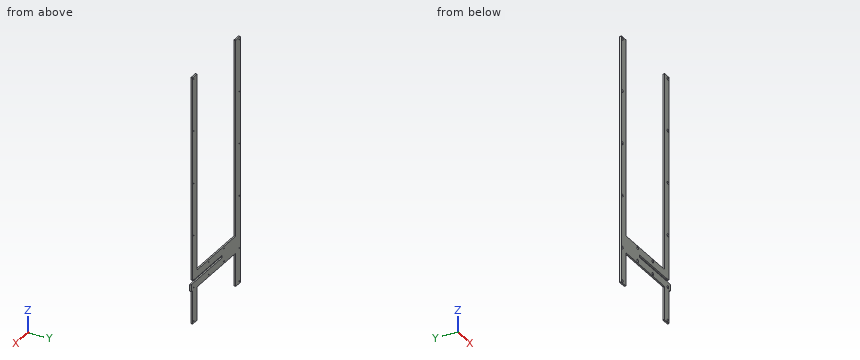
from build123d import *

# Parameters (mm, degrees)
BOSS_EXTRUDE1_DEPTH                                 = 9.525
SKETCH4_W                                           = 50.8
SKETCH4_H                                           = 200
BOSS_EXTRUDE2_DEPTH                                 = 9.525
CSK_FOR_1_4_FLAT_HEAD_MACHINE_SCREW_100_D           = 6.7564
CSK_FOR_1_4_FLAT_HEAD_MACHINE_SCREW_100_CSINK_D     = 17.6447958
CSK_FOR_1_4_FLAT_HEAD_MACHINE_SCREW_100_CSINK_ANGLE = 100
LPATTERN3_COUNT                                     = 2
LPATTERN3_PITCH                                     = 491.2
LPATTERN3_COUNT_DIR2                                = 5
LPATTERN3_PITCH_DIR2                                = 313.05
LPATTERN2_COUNT                                     = 3
LPATTERN2_PITCH                                     = 163.733333333
LPATTERN2_COUNT_DIR2                                = 2
LPATTERN2_PITCH_DIR2                                = 76.2
CSK_FOR_1_4_FLAT_HEAD_MACHINE_SCREW_2_D             = 6.7564
CSK_FOR_1_4_FLAT_HEAD_MACHINE_SCREW_2_CSINK_D       = 17.6447958
CSK_FOR_1_4_FLAT_HEAD_MACHINE_SCREW_2_CSINK_ANGLE   = 100
FILLET1_R                                           = 3.175
FILLET2_R                                           = 3.175


with BuildPart() as part:
    # Sketch1 → Boss-Extrude1 (new body)
    with BuildSketch(Plane(origin=(0, 0, 0), x_dir=(1, 0, 0), z_dir=(0, 1, 0))):
        Polygon((-258.3, 0), (-207.5, 0), (-207.5, 1176), (207.5, 1176), (207.5, 0), (258.3, 0), (258.3, 1215.514856628), (230.3, 1219.45), (-61.7, 1219.45), (-61.7, 1234.15), (271.3, 1234.15), (271.3, 1277.6), (-258.3, 1277.6), align=None)
    extrude(amount=BOSS_EXTRUDE1_DEPTH)

    # Sketch4 → Boss-Extrude2 (add)
    with BuildSketch(Plane.XZ):
        with Locations((-232.9, -1377.6)):
            Rectangle(SKETCH4_W, SKETCH4_H)
        with Locations((232.9, -1377.6)):
            Rectangle(SKETCH4_W, SKETCH4_H)
    extrude(amount=-BOSS_EXTRUDE2_DEPTH)

    # CSK for 1_4 Flat Head Machine Screw _100 (through all)
    with Locations(Plane.XZ):
        with Locations((-245.6, -1264.9)):
            csk_for_1_4_flat_head_machine_screw_100 = CounterSinkHole(CSK_FOR_1_4_FLAT_HEAD_MACHINE_SCREW_100_D / 2, CSK_FOR_1_4_FLAT_HEAD_MACHINE_SCREW_100_CSINK_D / 2, counter_sink_angle=CSK_FOR_1_4_FLAT_HEAD_MACHINE_SCREW_100_CSINK_ANGLE)

    # LPattern3: CSK for 1_4 Flat Head Machine Screw _100 2 × 5
    with Locations(*[(i * LPATTERN3_PITCH, 0, j * LPATTERN3_PITCH_DIR2) for i in range(LPATTERN3_COUNT) for j in range(LPATTERN3_COUNT_DIR2) if (i, j) != (0, 0)]):
        add(csk_for_1_4_flat_head_machine_screw_100, mode=Mode.SUBTRACT)

    # LPattern2: CSK for 1_4 Flat Head Machine Screw _100 3 × 2, 1 skipped
    with Locations(*[(i * LPATTERN2_PITCH, 0, j * LPATTERN2_PITCH_DIR2) for i in range(LPATTERN2_COUNT) for j in range(LPATTERN2_COUNT_DIR2) if (i, j) not in ((0, 0), (0, 1))]):
        add(csk_for_1_4_flat_head_machine_screw_100, mode=Mode.SUBTRACT)

    # CSK for 1_4 Flat Head Machine Screw  2 (through all)
    with Locations(Plane.XZ):
        with Locations((-245.6, -1464.9)):
            csk_for_1_4_flat_head_machine_screw_2 = CounterSinkHole(CSK_FOR_1_4_FLAT_HEAD_MACHINE_SCREW_2_D / 2, CSK_FOR_1_4_FLAT_HEAD_MACHINE_SCREW_2_CSINK_D / 2, counter_sink_angle=CSK_FOR_1_4_FLAT_HEAD_MACHINE_SCREW_2_CSINK_ANGLE)

    # Mirror1: CSK for 1_4 Flat Head Machine Screw  2 across plane
    add(csk_for_1_4_flat_head_machine_screw_2.mirror(Plane(origin=(0, 0, 0), x_dir=(0, 0, 1), z_dir=(1, 0, 0))), mode=Mode.SUBTRACT)

    # Fillet1
    fillet1_edges = [part.edges().sort_by_distance(p)[0] for p in [
        (258.3, 4.7625, 0),
        (207.5, 4.7625, 0),
        (-207.5, 4.7625, 0),
        (-258.3, 4.7625, 0),
        (207.5, 4.7625, -1176),
        (-207.5, 4.7625, -1176),
        (258.3, 4.7625, -1215.514856628),
        (271.3, 4.7625, -1234.15),
        (271.3, 4.7625, -1277.6),
        (-61.7, 4.7625, -1219.45),
        (-61.7, 4.7625, -1234.15),
    ]]
    fillet(fillet1_edges, radius=FILLET1_R)

    # Fillet2
    fillet2_edges = [part.edges().sort_by_distance(p)[0] for p in [
        (207.5, 4.7625, -1477.6),
        (258.3, 4.7625, -1477.6),
        (-258.3, 4.7625, -1477.6),
        (-207.5, 4.7625, -1477.6),
        (-207.5, 4.7625, -1277.6),
        (207.5, 4.7625, -1277.6),
        (258.3, 4.7625, -1277.6),
    ]]
    fillet(fillet2_edges, radius=FILLET2_R)


solid = part.part
The listing builds one solid part. Answer for the finished solid, in the listing's coordinates (mm). Round coordinates to 2 decimals unless told otherwise and drop trailing zeros. Write each loop counter-clockwise with the first axis right and the second up, starting at its lowest first coordinate (ties: lowest second). Pieces come first, ordered by that corner, then holes. Notation, with made-up numbers: (-12.5, -1.75) - (29.5, -1.75) arc R23 cw to (29.5, 14.25) - close; hole circle Ø2 at (46.5, 12.5). An arc over 180 degrees is marked (long way). Use a Markdown table: item, result. Add a question column.
1. The part is cut by section C-C (x = -174). Write down the section's boundary in (y, z) (3 decimals).
2. The part is cut by section A-A (z = -288). Write down the section's boundary in (x, y) (3 decimals).
3. Consider line 1 (X direction, y = 8.15, z = -325.75); line 2 (X direction, y = 6.15, z = -1188.7); line 3 (X direction, y = 5, z = -1167). Determine where each line is inside the solid, lowest interval first.
4. The part is cut by section D-D (y = 2). Give the number of separate pieces and of enclosed holes in the cut face, and give its area (3 significant figures).
5. The part is cut by section B-B (x = 29). Write down the section's boundary in (y, z) (3 decimals), and give its area (3 significant figures).
6. Flat-ended cylindrical pins translate along their axes: P1, Ø5, axis at y = 6, z = -1362, coming from the +X side; P2, Ø3.5, axis at x = 265, y = 3, coming from the -Z side; P3, Ø5, axis at x = 42.5, y = 6.5, coming from the +Z side. Find the tip coordinate at first contact, or state that the pin passes through.
Reported:
| question | item | result |
|---|---|---|
| 1 | outline | (0, -1277.6) - (9.525, -1277.6) - (9.525, -1176) - (0, -1176) - close |
| 2 | outline | (-258.3, 0) - (-207.5, 0) - (-207.5, 9.525) - (-258.3, 9.525) - close; (207.5, 0) - (258.3, 0) - (258.3, 9.525) - (207.5, 9.525) - close |
| 3 | line 1 | -258.3 to -248.98, -242.22 to -207.5, 207.5 to 242.22, 248.98 to 258.3 |
| 3 | line 2 | -258.3 to -85.24, -78.49 to 78.49, 85.24 to 258.3 |
| 3 | line 3 | -258.3 to -207.5, 207.5 to 258.3 |
| 4 | separate pieces | 1 |
| 4 | enclosed holes | 16 |
| 4 | area | 186,000 mm^2 |
| 5 | outline | (0, -1277.6) - (9.525, -1277.6) - (9.525, -1234.15) - (0, -1234.15) - close; (0, -1219.45) - (9.525, -1219.45) - (9.525, -1176) - (0, -1176) - close |
| 5 | area | 828 mm^2 |
| 6 | P1 | x = 258.3 |
| 6 | P2 | z = -1277.6 |
| 6 | P3 | z = -1176 |
